```python
from build123d import *

# Parameters (mm, degrees)
SKETCH1_R           = 1.75
BOSS_EXTRUDE1_DEPTH = 3.3
SKETCH3_R           = 4.3
BOSS_EXTRUDE3_DEPTH = 3


with BuildPart() as part:
    # Sketch1 → Boss-Extrude1 (new body)
    with BuildSketch(Plane.XY):
        with BuildLine():
            ThreePointArc((-51.5, -14.365), (-58.360069791, -6.024698512), (-67.867206803, -11.146761798))
            ThreePointArc((-67.867206803, -11.146761798), (-68.49399131, -14.045450902), (-68.08677112, -16.983039888))
            ThreePointArc((-68.08677112, -16.983039888), (-63.218238202, -22.232206803), (-56.066588393, -21.900135907))
            ThreePointArc((-56.066588393, -21.900135907), (-53.717281627, -20.090159373), (-52.132793197, -17.583238202))
            ThreePointArc((-52.132793197, -17.583238202), (-51.659698512, -16.004930209), (-51.5, -14.365))
        make_face()
        with Locations((-60, -14.365)):
            Circle(SKETCH1_R, mode=Mode.SUBTRACT)
        with BuildLine():
            ThreePointArc((-68.08677112, -16.983039888), (-68.49399131, -14.045450902), (-67.867206803, -11.146761798))
            Line((-67.867206803, -11.146761798), (-69.943886559, -16.223349695))
            Line((-69.943886559, -16.223349695), (-68.08677112, -16.983039888))
        make_face()
        with BuildLine():
            Line((-68.08677112, -16.983039888), (-69.943886559, -16.223349695))
            Line((-69.943886559, -16.223349695), (-80.356366151, -11.963916781))
            Line((-80.356366151, -11.963916781), (-86.414226296, -26.772776645))
            Line((-86.414226296, -26.772776645), (-49.854853507, -41.728118878))
            Line((-49.854853507, -41.728118878), (-43.103796568, -25.224691306))
            Line((-43.103796568, -25.224691306), (-52.547252782, -23.339790487))
            Line((-52.547252782, -23.339790487), (-54.209472954, -22.659826099))
            Line((-54.209472954, -22.659826099), (-56.066588393, -21.900135907))
            ThreePointArc((-56.066588393, -21.900135907), (-63.218238202, -22.232206803), (-68.08677112, -16.983039888))
        make_face()
        with Locations((-51.222303707, -32.525261715)):
            Circle(SKETCH1_R, mode=Mode.SUBTRACT)
        with Locations((-78.988915951, -21.166773943)):
            Circle(SKETCH1_R, mode=Mode.SUBTRACT)
        with BuildLine():
            Line((-54.209472954, -22.659826099), (-52.132793197, -17.583238202))
            ThreePointArc((-52.132793197, -17.583238202), (-53.717281627, -20.090159373), (-56.066588393, -21.900135907))
            Line((-56.066588393, -21.900135907), (-54.209472954, -22.659826099))
        make_face()
    extrude(amount=BOSS_EXTRUDE1_DEPTH)

    # Sketch3 → Boss-Extrude3 (add)
    with BuildSketch(Plane.XY.offset(3.3)):
        with Locations((-78.988915951, -21.166773943)):
            Circle(SKETCH3_R)
        Polygon((-75.785301718, -20.730667104), (-77.764788436, -18.174309213), (-80.96840267, -18.610416053), (-82.192530185, -21.602880783), (-80.213043466, -24.159238673), (-77.009429233, -23.723131834), align=None, mode=Mode.SUBTRACT)
        with Locations((-60, -14.365)):
            Circle(SKETCH3_R)
        Polygon((-63.203614234, -14.80110684), (-61.224127515, -17.35746473), (-58.020513281, -16.92135789), (-56.796385766, -13.92889316), (-58.775872485, -11.37253527), (-61.979486719, -11.80864211), align=None, mode=Mode.SUBTRACT)
        with Locations((-51.222303707, -32.525261715)):
            Circle(SKETCH3_R)
        Polygon((-54.42591794, -32.961368555), (-52.446431222, -35.517726445), (-49.242816988, -35.081619606), (-48.018689473, -32.089154876), (-49.998176192, -29.532796985), (-53.201790425, -29.968903825), align=None, mode=Mode.SUBTRACT)
    extrude(amount=BOSS_EXTRUDE3_DEPTH)


solid = part.part
```
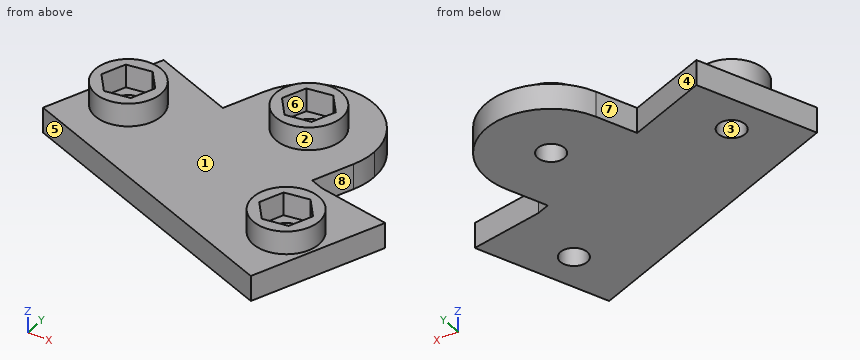
Work out the finished part from the listing and answer in its coordinate system (mm). Face numbers are marked on the shaded views. A direction names the side the tool comes from. Round coordinates to 2 decimals unless told otherwise and drop trailing zeros. Write each loop counter-clockwise with the first axis right and the second up, starting at its lowest first coordinate (ties: lowest second). Pieces come first, ordered by that corner, then holes.
1) Determine the mould class of the marked faces 1, 2, 3 and 4 for opening direction Y: pulls with the +Y half, pulls with the -Y half, needs draft (parallel to the pull), parting line crosses it, or undercut.
2) A cutting plane is placed at C-C on z = 2.5. Determine the outline of the cut face in (x, y) (3 decimals), and give its area (3 significant figures).
3) Which of the six approach directions +Z, -Z, +X, -X, +Y, -Y give full straight-line access (tool end or side, diameter ignored) to the marked faces 5, 6, 7 and 8?
4) Flat-ended cylindrical pins translate along their axes: P1, Ø2, axis at x = -51.22, y = -32.53, coming from the -Z side; P2, Ø1, axis at x = -53, y = -25, coming from the +Z side; P3, Ø1.5, axis at y = -18, z = 3, coming from the +X side. Find the tip coordinate at first contact, or state that the pin passes through.
5) A cutting plane is placed at A-A on z = 5. Determine the outline of the cut face in (x, y) (3 decimals), and give its area (3 significant figures).
6) Consider probe 1 along X at (y, z) = (-32, 5.5); probe 2 along Y at (x, z) = (-52.5, 1.25) (3 decimals); probe 3 along Z at (x, y) = (-59, -33.5). Determine where each line is inside the solid, lowest interval first.
7) A cutting plane is placed at B-B on x = -60. Determine the outline of the cut face in (y, z) (3 decimals).
8) A cutting plane is placed at D-D on x = -81.5. Determine the outline of the cut face in (y, z), and give its area (3 significant figures).
Entries:
1. face 1: needs draft
1. face 2: parting line crosses it
1. face 3: undercut
1. face 4: pulls with the +Y half
2. outline: (-86.414, -26.773) - (-49.855, -41.728) - (-43.104, -25.225) - (-52.547, -23.34) - (-54.209, -22.66) - (-52.133, -17.583) arc R8.5 ccw to (-67.867, -11.147) - (-69.944, -16.223) - (-80.356, -11.964) - close; hole circle Ø3.5 at (-78.989, -21.167); hole circle Ø3.5 at (-60, -14.365); hole circle Ø3.5 at (-51.222, -32.525)
2. area: 819 mm2
3. face 5: +Z, -Z, -X, -Y
3. face 6: +Z
3. face 7: +Z, -Z, +Y
3. face 8: +Z, -Z, +X
4. P1: passes through
4. P2: stops at z = 3.3
4. P3: stops at x = -52
5. outline: circle Ø8.6 at (-78.989, -21.167); circle Ø8.6 at (-60, -14.365); circle Ø8.6 at (-51.222, -32.525); hole (-82.193, -21.603) - (-80.213, -24.159) - (-77.009, -23.723) - (-75.785, -20.731) - (-77.765, -18.174) - (-80.968, -18.61) - close; hole (-63.204, -14.801) - (-61.224, -17.357) - (-58.021, -16.921) - (-56.796, -13.929) - (-58.776, -11.373) - (-61.979, -11.809) - close; hole (-54.426, -32.961) - (-52.446, -35.518) - (-49.243, -35.082) - (-48.019, -32.089) - (-49.998, -29.533) - (-53.202, -29.969) - close
5. area: 92.8 mm2
6. probe 1: x = -55.49 to -54.03, -48.09 to -46.95
6. probe 2: y = -40.646 to -33.721, -31.329 to -23.349, -18.481 to -10.365
6. probe 3: z = 0 to 3.3
7. outline: (-37.578, 0) - (-16.115, 0) - (-16.115, 3.3) - (-17.191, 3.3) - (-17.191, 6.3) - (-18.665, 6.3) - (-18.665, 3.3) - (-37.578, 3.3) - close; (-12.615, 0) - (-5.865, 0) - (-5.865, 3.3) - (-10.065, 3.3) - (-10.065, 6.3) - (-11.539, 6.3) - (-11.539, 3.3) - (-12.615, 3.3) - close
8. outline: (-28.78, 0) - (-14.76, 0) - (-14.76, 3.3) - (-17.68, 3.3) - (-17.68, 6.3) - (-19.91, 6.3) - (-19.91, 3.3) - (-22.5, 3.3) - (-22.5, 6.3) - (-24.66, 6.3) - (-24.66, 3.3) - (-28.78, 3.3) - close
8. area: 59.5 mm2
